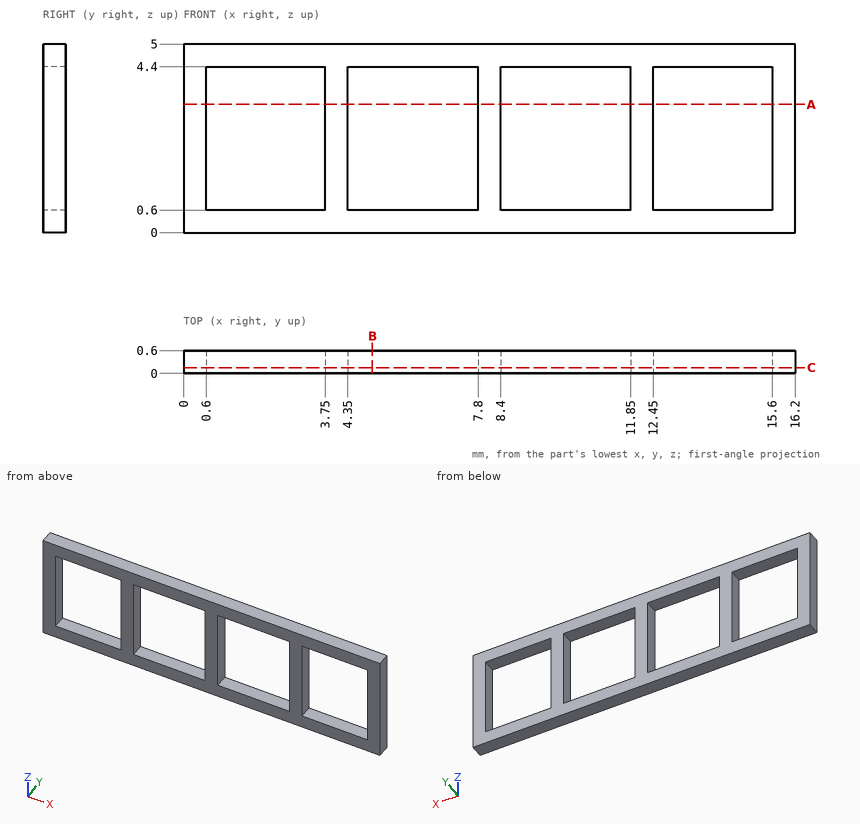
Verification items for this drawing (mm, ordinates from the low corner). Give positions to 0.01 mm unless a question says otherwise; leave off trailing zeros. Loops run counter-clockwise (first coordinate to the right, second up) from the corner with the lowest first, then second, coordinate; pieces in that order, holes last. Notation, with made-up numbers: M -27.5,49.5 L 25.5,49.5 A16 cw 25.5,60.5 Z; hole C 81,32.5 d7. An arc over 180 degrees is marked long. Write item = value, one per line.
(1) Sectioned sample at A-A, the plane z = 3.4. Record the cut outline in (x, y).
Answer below:
outline = M 0,0 L 0.6,0 L 0.6,0.6 L 0,0.6 Z; M 3.75,0 L 4.35,0 L 4.35,0.6 L 3.75,0.6 Z; M 7.8,0 L 8.4,0 L 8.4,0.6 L 7.8,0.6 Z; M 11.85,0 L 12.45,0 L 12.45,0.6 L 11.85,0.6 Z; M 15.6,0 L 16.2,0 L 16.2,0.6 L 15.6,0.6 Z
(2) Sectioned sample at C-C, the plane y = 0.15. Record the cut outline in (x, z), plus the area to 3 significant figures.
Answer below:
outline = M 0,0 L 16.2,0 L 16.2,5 L 0,5 Z; hole M 0.6,0.6 L 3.75,0.6 L 3.75,4.4 L 0.6,4.4 Z; hole M 4.35,0.6 L 7.8,0.6 L 7.8,4.4 L 4.35,4.4 Z; hole M 8.4,0.6 L 11.85,0.6 L 11.85,4.4 L 8.4,4.4 Z; hole M 12.45,0.6 L 15.6,0.6 L 15.6,4.4 L 12.45,4.4 Z
area = 30.8 mm2
(3) Sectioned sample at B-B, the plane x = 5. Record the cut outline in (y, z).
Answer below:
outline = M 0,0 L 0.6,0 L 0.6,0.6 L 0,0.6 Z; M 0,4.4 L 0.6,4.4 L 0.6,5 L 0,5 Z
(4) Material ranges on line 1 (X direction, y = 0.3, z = 2.35); line 2 (Z direction, x = 5.25, y = 0.15), recorded low to high. Write a range as [from, to].
Answer below:
line_1 = [0, 0.6], [3.75, 4.35], [7.8, 8.4], [11.85, 12.45], [15.6, 16.2]
line_2 = [0, 0.6], [4.4, 5]
